from build123d import *

# Parameters (mm, degrees)
RESSALTO_EXTRUS_O1_DEPTH = 15
ESBO_O2_R                = 1
CORTE_EXTRUS_O1_DEPTH    = 41.926763859
FILETE1_R                = 3


with BuildPart() as part:
    # Esbo_o1 → Ressalto-extrus_o1 (new body)
    with BuildSketch(Plane(origin=(0, 0, 0), x_dir=(1, 0, 0), z_dir=(0, 1, 0))):
        with BuildLine():
            Line((0, 15), (0, 0))
            Line((0, 0), (35, 0))
            Line((35, 0), (35, 15))
            Line((35, 15), (30, 15))
            ThreePointArc((30, 15), (17.5, 2.5), (5, 15))
            Line((5, 15), (0, 15))
        make_face()
    extrude(amount=RESSALTO_EXTRUS_O1_DEPTH)

    # Esbo_o2 → Corte-extrus_o1 (cut, through all)
    with BuildSketch(Plane(origin=(0, 0, -15), x_dir=(-1, 0, 0), z_dir=(0, 0, -1))):
        with Locations((-32.5, 12.5)):
            Circle(ESBO_O2_R)
        with Locations(Location((-32.5, 2.5, 0), (0, 0, 180))):
            Circle(ESBO_O2_R)
        with Locations((-2.5, 2.5)):
            Circle(ESBO_O2_R)
        with Locations(Location((-2.5, 12.5, 0), (0, 0, 180))):
            Circle(ESBO_O2_R)
    extrude(amount=-CORTE_EXTRUS_O1_DEPTH, mode=Mode.SUBTRACT)

    # Filete1
    filete1_edges = [part.edges().sort_by_distance(p)[0] for p in [
        (0, 15, -7.5),
        (35, 15, -7.5),
        (35, 0, -7.5),
        (0, 0, -7.5),
    ]]
    fillet(filete1_edges, radius=FILETE1_R)


solid = part.part
Read the model definition and answer for the solid it produces. Units are mm, in the model's axes. Coordinates: 2 decimals unless noted, no trailing zeros. Loops run counter-clockwise (first coordinate to the right, second up) from the corner with the lowest first, then second, coordinate; pieces in that order, holes last. Notation, with made-up numbers: (88, -3.75) -> (120, -3.75) arc R17 cw to (120, 27.25) -> close; hole circle Ø2 at (82.5, 4.5). An arc over 180 degrees is marked (long way). Answer in a Markdown table with one row per item.
Item 1: A cutting plane is placed at A-A on z = -12.5. Determine the outline of the cut face in (x, y), plus the area to 3 significant figures.
Returned:
| item | result |
|---|---|
| outline | (0, 3) arc R3 ccw to (3, 0) -> (5.25, 0) -> (5.25, 15) -> (3, 15) arc R3 ccw to (0, 12) -> close; (29.75, 0) -> (32, 0) arc R3 ccw to (35, 3) -> (35, 12) arc R3 ccw to (32, 15) -> (29.75, 15) -> close; hole circle Ø2 at (2.5, 2.5); hole circle Ø2 at (2.5, 12.5); hole circle Ø2 at (32.5, 2.5); hole circle Ø2 at (32.5, 12.5) |
| area | 137 mm^2 |
Item 2: A cutting plane is placed at D-D on z = -2. Determine the outline of the cut face in (x, y), plus the area to 3 significant figures.
Returned:
| item | result |
|---|---|
| outline | (0, 3) arc R3 ccw to (3, 0) -> (32, 0) arc R3 ccw to (35, 3) -> (35, 12) arc R3 ccw to (32, 15) -> (3, 15) arc R3 ccw to (0, 12) -> close; hole circle Ø2 at (2.5, 2.5); hole circle Ø2 at (2.5, 12.5); hole circle Ø2 at (32.5, 2.5); hole circle Ø2 at (32.5, 12.5) |
| area | 505 mm^2 |
Item 3: A cutting plane is placed at C-C on x = 32.5. Determine the outline of the cut face in (y, z).
Returned:
| item | result |
|---|---|
| outline | (0.04, -15) -> (1.5, -15) -> (1.5, 0) -> (0.04, 0) -> close; (3.5, -15) -> (11.5, -15) -> (11.5, 0) -> (3.5, 0) -> close; (13.5, -15) -> (14.96, -15) -> (14.96, 0) -> (13.5, 0) -> close |
Item 4: A cutting plane is placed at B-B on y = 2.5. Determine the outline of the cut face in (x, z), plus the area to 3 significant figures.
Returned:
| item | result |
|---|---|
| outline | (0.04, -15) -> (1.5, -15) -> (1.5, 0) -> (0.04, 0) -> close; (3.5, -15) -> (5, -15) arc R12.5 cw to (30, -15) -> (31.5, -15) -> (31.5, 0) -> (3.5, 0) -> close; (33.5, -15) -> (34.96, -15) -> (34.96, 0) -> (33.5, 0) -> close |
| area | 218 mm^2 |
Item 5: Straight lines are drawn through the part: line 1 along Y through (x, z) = (32, -5.25); line 2 along Y through (x, z) = (32.5, -6); line 3 along X through (y, z) = (3, -10.25). For each, find the intervals that lie inside material, in ascending order. Write a range as [from, to].
Returned:
| item | result |
|---|---|
| line 1 | y = [0, 1.63], [3.37, 11.63], [13.37, 15] |
| line 2 | y = [0.04, 1.5], [3.5, 11.5], [13.5, 14.96] |
| line 3 | x = [0, 1.63], [3.37, 5.94], [29.06, 31.63], [33.37, 35] |
Item 6: For a pull along Y with two mould halves and no side action, classify faces 1 (the cylindrical face through (0.86, 14.1, -7.4)), 2 (the flat face through (17, 7, 0)), 3 (the cylindrical face through (3.5, 2.5, -7.6)) as released by +Y, released by -Y, zero draft, split by the parting line, or undercut.
Returned:
| item | result |
|---|---|
| face 1 | released by +Y |
| face 2 | zero draft |
| face 3 | undercut |
